Can you work these out from the model? Positions are in its coordinate system, mm. Face numbers are marked on the shaded views. A direction names the side the tool comes from. Give positions to 0.01 mm unless a question says otherwise; leave off trailing zeros. Order: outer loops, then holes, each group sorted by start corner. A loop starts at its lowest first (then second) coordinate and runs counter-clockwise, first axis right, second up. Notation, with made-up numbers: M -24,15 L 3,15 A14 cw 3,38 Z; hole C 15.25,0.25 d9. An arc over 180 degrees is marked long. One line per question, with ' | ' between items. Start each with the question number.
1) Please list where these lines run through material, in increasing order: line 1 along X through (y, z) = (7, -2.5); line 2 along Y through (x, z) = (0, 1.5); line 3 along Y through (x, z) = (22.5, -7.75). Write a range as [from, to].
2) For the marked faces 5, 6 and 7, which set-ups out of +Z, -Z, +X, -X, +Y, -Y let a thin tool reach every point of the face, with its end or its side?
3) Thinking about a two-plate mould opening in X: for the marked faces 1, 2, 3 and 4, which applies, +X half, -X half, draft (parallel to the pull), parting line (faces both ways), or undercut?
4) If we section it at B-B, the plane z = 3: Please give me the cut outline in (x, y), plus the area to 3 significant figures.
5) If we section it at A-A, the plane x = 0: Please give me the cut outline in (y, z), plus the area to 3 significant figures.
6) If we section it at D-D, the plane x = -30: Please give me the cut outline in (y, z), plus the area to 3 significant figures.
7) If we section it at C-C, the plane z = -13: Please give me the cut outline in (x, y).
8) I'm going to push flat-ended pins straight in: pin 1 Ø6 at (x, z) = (-24, 8) entering from +Y; pin 2 Ø1.5 at (y, z) = (13.5, -1.5) entering from +X; pin 3 Ø16 at (x, y) = (0, 29) entering from +Z; pin 4 Ø5 at (y, z) = (39.5, -9.5) entering from -X. Where does each tip first touch, or does it pass through?
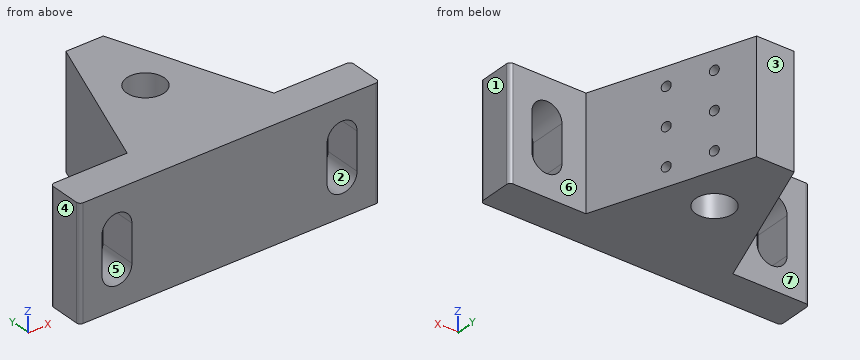
```python
from build123d import *

# Parameters (mm, degrees)
BASE_EXTRUDE_DEPTH   = 15
SLOT_CUT_DEPTH       = 66.76473219
SKETCH5_R            = 5
GUIDE_HOLE_DEPTH     = 71.710678119
LPATTERN1_COUNT      = 3
LPATTERN1_PITCH      = 10
LPATTERN1_COUNT_DIR2 = 2
LPATTERN1_PITCH_DIR2 = 12
FILLET1_R            = 1


with BuildPart() as part:
    # Sketch2 → Base Extrude (new, symmetric)
    with BuildSketch(Plane.XY):
        Polygon((-40, 0), (40, 0), (40, 10), (19.558809371, 10), (5, 50), (-5, 50), (-19.558809371, 10), (-40, 10), align=None)
    extrude(amount=BASE_EXTRUDE_DEPTH, both=True)

    # Sketch4 → Slot Cut (cut, through all)
    with BuildSketch(Plane(origin=(0, 0, 0), x_dir=(1, 0, 0), z_dir=(0, 1, 0))):
        with BuildLine():
            Line((26, -5), (26, 5))
            ThreePointArc((26, 5), (30, 9), (34, 5))
            Line((34, 5), (34, -5))
            ThreePointArc((34, -5), (30, -9), (26, -5))
        make_face()
    slot_cut = extrude(amount=SLOT_CUT_DEPTH, mode=Mode.SUBTRACT)

    # Mirror1: Slot Cut across plane
    add(slot_cut.mirror(Plane(origin=(0, 0, 0), x_dir=(0, 0, 1), z_dir=(1, 0, 0))), mode=Mode.SUBTRACT)

    # Sketch5 → Guide Hole (cut, through all)
    with BuildSketch(Plane.XY.offset(15)):
        with Locations((0, 29)):
            Circle(SKETCH5_R)
    extrude(amount=-GUIDE_HOLE_DEPTH, mode=Mode.SUBTRACT)

    # Sketch10 → M3x0.5 Tapped Hole2 (revolve, cut)
    with BuildSketch(Plane(origin=(12.718406504, 28.793852416, 10), x_dir=(-0.3420201433256662, 0.9396926207859093, 0), z_dir=(0, 0, 1))):
        Polygon((0, 0), (0, 8.251075774), (1.25, 7.5), (1.25, 0), align=None)
    m3x0_5_tapped_hole2 = revolve(axis=Axis((18.685454646, 30.965680326, 10), (-0.9396926207859093, -0.34202014332566616, 0)), mode=Mode.SUBTRACT)

    # LPattern1: M3x0.5 Tapped Hole2 3 × 2
    with Locations(*[Vector(0, 0, -1) * (i * LPATTERN1_PITCH) + Vector(-0.34202014332566616, 0.9396926207859094, 0) * (j * LPATTERN1_PITCH_DIR2) for i in range(LPATTERN1_COUNT) for j in range(LPATTERN1_COUNT_DIR2) if (i, j) != (0, 0)]):
        add(m3x0_5_tapped_hole2, mode=Mode.SUBTRACT)

    # Fillet1
    fillet1_edges = [part.edges().sort_by_distance(p)[0] for p in [
        (40, 0, 0),
        (-40, 0, 0),
        (-40, 10, 0),
        (40, 10, 0),
    ]]
    fillet(fillet1_edges, radius=FILLET1_R)


solid = part.part
```
Results found:
1) line 1: x = [-40, -34], [-26, 26], [34, 40] | line 2: y = [0, 24], [34, 50] | line 3: y = [0, 10]
2) face 5: +Y, -Y | face 6: +Z, -Z, +X, +Y | face 7: +Z, -Z, -X, +Y
3) face 1: +X half | face 2: undercut | face 3: draft | face 4: -X half
4) outline: M -40,1 A1 ccw -39,0 L -34,0 L -34,10 L -39,10 A1 ccw -40,9 Z; M -26,0 L 26,0 L 26,10 L 19.56,10 L 5,50 L -5,50 L -19.56,10 L -26,10 Z; M 34,0 L 39,0 A1 ccw 40,1 L 40,9 A1 ccw 39,10 L 34,10 Z; hole C 0,29 d10 | area: 1,540 mm²
5) outline: M 0,-15 L 24,-15 L 24,15 L 0,15 Z; M 34,-15 L 50,-15 L 50,15 L 34,15 Z | area: 1,200 mm²
6) outline: M 0,-15 L 10,-15 L 10,-9 L 0,-9 Z; M 0,9 L 10,9 L 10,15 L 0,15 Z | area: 120 mm²
7) outline: M -40,1 A1 ccw -39,0 L 39,0 A1 ccw 40,1 L 40,9 A1 ccw 39,10 L 19.56,10 L 5,50 L -5,50 L -19.56,10 L -39,10 A1 ccw -40,9 Z; hole C 0,29 d10
8) pin 1: stops at y = 10 | pin 2: stops at x = 18.56 | pin 3: stops at z = 15 | pin 4: stops at x = -9.73
